Could you check a few things on this model? Use its own coordinates, in mm. Give positions to 0.01 mm unless a question says otherwise; leave off trailing zeros. Loops run counter-clockwise (first coordinate to the right, second up) from the corner with the lowest first, then second, coordinate; pieces in that order, holes last. Notation, with made-up numbers: (60, 39.25) - (74, 39.25) arc R35 ccw to (74, 71.25) - close; hole circle Ø7 at (43.5, -18.75). An arc over 180 degrees is marked (long way). Write each question's results on one line, items separated by ' | '. Start each with the question number.
(1) Suppose I cut it at A-A (x = 33). Please give me the cut outline in (y, z).
(2) Suppose I cut it at B-B (z = 13.5). Please give me the cut outline in (x, y).
(3) I need wall thicknesses on line 1 (Y direction, x = 6.5, z = 24.25); line 2 (Y direction, x = 6.5, z = 9); line 3 (Z direction, x = 33.5, y = 15.75). Which ranges of each line are inside material? Lowest first, please.
(4) For pin 1 (6 mm diameter, centred on y = -1.5, z = 21, fed in from -X); pin 2 (13 mm diameter, centred on x = 17.5, z = 17.5, fed in from -Y), each with a flat end and sliding along its axis, tell me the tip position at first contact or that it passes through.
from build123d import *

# Parameters (mm, degrees)
SKETCH1_W           = 45
SKETCH1_H           = 16.5
BOSS_EXTRUDE1_DEPTH = 28
SKETCH2_R           = 0.3
BOSS_EXTRUDE2_DEPTH = 4
FILLET1_R           = 1


with BuildPart() as part:
    # Sketch1 → Boss-Extrude1 (new body)
    with BuildSketch(Plane.XY):
        with Locations((22.5, 8.25)):
            Rectangle(SKETCH1_W, SKETCH1_H)
    extrude(amount=BOSS_EXTRUDE1_DEPTH)

    # Sketch2 → Boss-Extrude2 (add)
    with BuildSketch(Plane(origin=(0, 0, 0), x_dir=(-1, 0, 0), z_dir=(0, -1, 0))):
        with Locations(Location((-6, -19, 0), (0, 0, 270))):
            Circle(SKETCH2_R)
        with Locations(Location((-6, -9, 0), (0, 0, 270))):
            Circle(SKETCH2_R)
        with Locations(Location((-39, -24, 0), (0, 0, 270))):
            Circle(SKETCH2_R)
        with Locations(Location((-39, -4, 0), (0, 0, 270))):
            Circle(SKETCH2_R)
    extrude(amount=BOSS_EXTRUDE2_DEPTH)

    # Fillet1
    fillet1_edges = [part.edges().sort_by_distance(p)[0] for p in [
        (45, 8.25, 28),
        (22.5, 16.5, 28),
        (6, 0, 18.7),
        (6, 0, 8.7),
        (39, 0, 23.7),
        (39, 0, 3.7),
        (0, 8.25, 28),
        (22.5, 16.5, 0),
        (45, 8.25, 0),
        (22.5, 0, 0),
        (0, 8.25, 0),
        (22.5, 0, 28),
        (0, 16.5, 14),
        (45, 16.5, 14),
        (45, 0, 14),
        (0, 0, 14),
    ]]
    fillet(fillet1_edges, radius=FILLET1_R)


solid = part.part
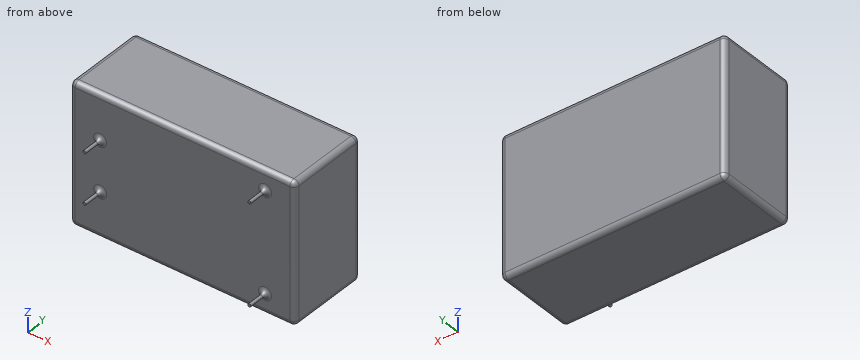
Output values:
1) outline: (0, 1) arc R1 ccw to (1, 0) - (15.5, 0) arc R1 ccw to (16.5, 1) - (16.5, 27) arc R1 ccw to (15.5, 28) - (1, 28) arc R1 ccw to (0, 27) - close
2) outline: (0, 1) arc R1 ccw to (1, 0) - (44, 0) arc R1 ccw to (45, 1) - (45, 15.5) arc R1 ccw to (44, 16.5) - (1, 16.5) arc R1 ccw to (0, 15.5) - close
3) line 1: 0 to 16.5 | line 2: -0.4 to 16.5 | line 3: 0.03 to 27.97
4) pin 1: x = 0 | pin 2: y = 0
